Part model, mm, in its own coordinate system. A direction names the side the tool comes from. Give positions to 0.01 mm unless a question says otherwise; leave off trailing zeros. Write each loop counter-clockwise with the first axis right and the second up, starting at its lowest first coordinate (ties: lowest second). Pieces come first, ordered by that corner, then holes. Notation, with made-up numbers: (-26.5, -18.75) - (-12.5, -18.75) arc R19 ccw to (-12.5, 4.25) - close; hole circle Ø8 at (-22.75, -15). An arc over 180 degrees is marked (long way). Answer in a Markdown table with one row per item. Add a question column.
1. Band-saw the part on D-D on z = 2.7. Write the cut outline in (x, y), plus the area to 3 significant figures.
2. Probe line 1 along Z through (x, y) = (-7, -9.25); line 2 along Y through (x, z) = (-16, 3.4); line 3 along Y through (x, z) = (-13.25, 4.5). List the from-to ranges inside material, lowest first.
3. Band-saw the part on C-C on z = 1.2. Write the cut outline in (x, y), plus the area to 3 significant figures.
4. Band-saw the part on A-A on y = -5.5. Write the cut outline in (x, z).
5. Which spindle directions (+Z, -Z, +X, -X, +Y, -Y) get a long thin tool onto all of the face, cutting with end or side? Do faces 5 (the flat face through (-8, -10.7, 2)), 6 (the flat face through (-10, -5, 0)). Say none if no direction does.
6. Pull direction Y, two halves, no side cores. Call faces 1 (the flat face through (-9, 0, 2)), 2 (the flat face through (-20.377, -5, 2)), 3 (the flat face through (-8, -11, 2)), 4 (the flat face through (-10, -6, 4.7)): released by +Y, released by -Y, zero draft, split by the parting line, or undercut.
7. Band-saw the part on B-B on x = -2.75. Write the cut outline in (y, z).
8. Drop a flat-ended pin along its axis: pin 1 Ø0.6 at (y, z) = (-0.5, 2.5) entering from -X. Give the stop position or say it passes through.
Autodesk Inventor part; units mm, degrees
ref_plane "Work Plane1" through (-16.877, -0.4, 5) normal (-0.6428, 0, 0.766) x (0, -1, 0)
ref_plane "Work Plane2" through (-16.877, -0.4, 0) normal (-0.6428, 0, -0.766) x (0, -1, 0)
ref_plane "YZ Plane" through (0, 0, 0) normal (1, 0, 0) x (0, 1, 0)
sketch "Sketch1" plane through (0, 0, 0) normal (0, 0, 1) x (1, 0, 0)
  line L0 (0, -11) -> (-16.777, -11)
  line L1 (-16.777, -11) -> (-16.777, -10.7)
  line L2 (-16.777, -10.7) -> (0, -10.7)
  line L3 (0, -10.7) -> (0, -11)
  line L4 (0, -0.3) -> (-16.777, -0.3)
  line L5 (-16.777, -0.3) -> (-16.777, 0)
  line L6 (-16.777, 0) -> (0, 0)
  line L7 (0, 0) -> (0, -0.3)
  line L8 (-20.377, -8.65) -> (-20.777, -8.65)
  line L9 (-20.777, -8.65) -> (-20.777, -2.35)
  line L10 (-20.777, -2.35) -> (-20.377, -2.35)
  line L11 (-20.377, -2.35) -> (-20.377, -8.65)
  line L12 (-20.377, -8.65) -> (-16.777, -10.7)
  line L13 (-16.777, -11) -> (-20.777, -8.65)
  line L14 (-20.777, -2.35) -> (-16.777, 0)
  line L15 (-20.377, -2.35) -> (-16.777, -0.3)
  dimension "d0" = 0.3
  dimension "d2" = 10.4
  dimension "d3" = 0.4
  dimension "d4" = 4
  dimension "d21" = 20.777
  dimension "d22" = 6.3
extrude "Extrusion1" add sketch "Sketch1" along normal blind 5
sketch "Sketch2" plane through (-16.777, -10.7, 0) normal (0, 1, 0) x (1, 0, 0)
  line L0 (4.777, -3.6) -> (4.377, -3.6)
  line L1 (4.377, -3.6) -> (4.377, -1.4)
  line L2 (4.377, -1.4) -> (4.777, -1.4)
  line L3 (4.777, -1.4) -> (4.777, -3.6)
  line L4 (4.777, -3.6) -> (4.777, -5) construction
  line L5 (16.777, -5) -> (0, -5) construction
  line L6 (4.777, -1.4) -> (4.777, 0) construction
  line L7 (16.777, 0) -> (0, 0) construction
  line L8 (16.777, 0) -> (16.777, -5) construction
  dimension "d9" = 0.4
  dimension "d10" = 1.4
  dimension "d11" = 12
extrude "Extrusion2" add sketch "Sketch2" along normal blind 0.5
sketch "Sketch3" plane through (-16.777, -0.3, 0) normal (0, -1, 0) x (1, 0, 0)
  line L0 (4.777, 1.4) -> (4.377, 1.4)
  line L1 (4.377, 1.4) -> (4.377, 3.6)
  line L2 (4.377, 3.6) -> (4.777, 3.6)
  line L3 (4.777, 3.6) -> (4.777, 1.4)
  point P0 (16.777, 0)
extrude "Extrusion3" add sketch "Sketch3" along normal blind 0.5
sketch "Sketch4" plane through (0, -0.3, 0) normal (1, 0, 0) x (0, 0, -1)
  line L0 (0, -10.4) -> (-5, -10.4)
  line L1 (0, 0) -> (-5, 0)
  line L2 (-5, -10.4) -> (-4.7, -10.4)
  line L3 (-4.7, -10.4) -> (-4.7, 0)
  line L4 (-4.7, 0) -> (-5, 0)
  line L5 (-5, 0) -> (-5, -10.4)
  line L6 (0, 0) -> (-0.3, 0)
  line L7 (-0.3, 0) -> (-0.3, -10.4)
  line L8 (-0.3, -10.4) -> (0, -10.4)
  line L9 (0, -10.4) -> (0, 0)
  point P0 (0, 0.3)
  point P1 (-0.3, 0)
  dimension "d16" = 0.3
  dimension "d17" = 0.3
extrude "Extrusion4" add sketch "Sketch4" against normal up to next contours L0 L7 L1 L9 | L0 L5 L1 L3
fillet "Fillet1" radius 0.4 18 edges at (-20.777, -5.5, 0) (-18.777, -9.825, 0) (-18.777, -9.825, 5) (-20.777, -5.5, 5) (-18.777, -1.175, 0) (-18.777, -1.175, 5) (-8.3885, 0, 5) (-8.3885, 0, 0) (-8.3885, -11, 5) (-8.3885, -11, 0) (-8.3885, -10.7, 0.3) (-16.777, -10.7, 2.5) (-20.377, -8.65, 2.5) (-20.377, -2.35, 2.5) (-16.777, -0.3, 2.5) (-8.3885, -0.3, 0.3) (-8.3885, -0.3, 4.7) (-8.3885, -10.7, 4.7)
sketch "Sketch5" plane through (0, 0, 5) normal (0, 0, 1) x (1, 0, 0)
  line L0 (0, -0.4) -> (-16.6682, -0.4)
  line L1 (-16.877, -0.4) -> (-16.877, -10.7)
  line L2 (-16.6711, -10.7) -> (0, -10.7)
  line L3 (-20.377, -8.4211) -> (-20.377, -2.5789)
  point P0 (0, 0)
  dimension "d23" = 3.5
ref_plane "Work Plane1" through (-16.877, -0.4, 5) normal (-0.6428, 0, 0.766) x (0, -1, 0)
sketch "Sketch6" plane through (0, 0, 0) normal (0, 0, -1) x (-1, 0, 0)
  line L0 (16.877, -0.4) -> (16.877, -10.7)
  point P0 (0, 0)
ref_plane "Work Plane2" through (-16.877, -0.4, 0) normal (-0.6428, 0, -0.766) x (0, -1, 0)
sketch "Sketch7" plane through (-16.877, -0.4, 5) normal (-0.6428, 0, 0.766) x (0, -1, 0)
  line L0 (0.35, 0.6) -> (9.85, 0.6)
  line L1 (9.85, 0.6) -> (9.85, 0)
  line L2 (9.85, 0) -> (0.35, 0)
  line L3 (0.35, 0) -> (0.35, 0.6)
  line L4 (0, 0) -> (10.3, 0)
  line L5 (-0.4, 12.6714) -> (-0.4, -0.1805) construction
  line L6 (10.6, -0.1805) -> (10.6, 12.6714) construction
  line L7 (0.35, 0.6) -> (-0.4, 0.6) construction
  line L8 (9.85, 0.6) -> (10.6, 0.6) construction
  point P0 (-0.4, 9.7146)
  dimension "d26" = 9.5
  dimension "d27" = 0.6
extrude "Extrusion5" cut sketch "Sketch7" against normal blind 3
sketch "Sketch8" plane through (-16.877, -0.4, 0) normal (-0.6428, 0, -0.766) x (0, -1, 0)
  line L0 (9.85, -0.6) -> (0.35, -0.6)
  line L1 (0.35, -0.6) -> (0.35, 0)
  line L2 (0.35, 0) -> (9.85, 0)
  line L3 (9.85, 0) -> (9.85, -0.6)
  line L4 (0, 0) -> (10.3, 0)
  line L5 (0.35, 3.2139) -> (0.35, 2.6139)
  line L6 (9.85, 2.6139) -> (9.85, 3.2139)
  line L7 (10.6, -12.6714) -> (10.6, 0.1805)
  line L8 (-0.4, 0.1805) -> (-0.4, -12.6714)
  line L9 (0.35, -0.6) -> (-0.4, -0.6) construction
  line L10 (9.85, -0.6) -> (10.6, -0.6) construction
  point P0 (-0.4, -12.9285)
  dimension "d30" = 9.5
  dimension "d31" = 0.6
extrude "Extrusion6" cut sketch "Sketch8" against normal blind 3
sketch "Sketch9" plane through (0, 0, 0) normal (0, 0, -1) x (-1, 0, 0)
  circle A0 centre (19.977, -7.6) radius 0.4
  line L0 (19.977, -2.1106) -> (19.977, -5.2) construction
  line L1 (20.777, -8.65) -> (20.777, -2.35)
  circle A1 centre (19.977, -6.2) radius 0.4
  circle A2 centre (19.977, -4.8) radius 0.4
  circle A3 centre (19.977, -3.4) radius 0.4
  circle A4 centre (17.777, -7.6) radius 0.4
  line L2 (17.777, -0.9242) -> (17.777, -5.2) construction
  circle A5 centre (17.777, -6.2) radius 0.4
  circle A6 centre (17.777, -4.8) radius 0.4
  circle A7 centre (17.777, -3.4) radius 0.4
  circle A8 centre (17.777, -9) radius 0.4
  circle A9 centre (17.777, -2) radius 0.4
  line L3 (19.977, -8) -> (19.977, -8.65) construction
  line L4 (20.777, -2.35) -> (16.777, 0)
  line L5 (20.777, -2.35) -> (20.777, -8.65)
  line L6 (20.777, -5.5) -> (17.4188, -5.5)
  line L7 (19.977, -5.5) -> (19.977, -5.8) construction
  line L8 (19.977, -5.8) -> (19.977, -8) construction
  line L9 (19.977, -5.2) -> (19.977, -5.5) construction
  line L10 (17.777, -5.8) -> (17.777, -10.129) construction
  line L11 (17.777, -5.5) -> (17.777, -5.8) construction
  line L12 (17.777, -5.2) -> (17.777, -5.5) construction
  line L13 (18.877, -9.1995) -> (18.877, -2.1819) construction
  circle A10 centre (18.877, -6.9) radius 0.4
  circle A11 centre (18.877, -5.5) radius 0.4
  circle A12 centre (18.877, -4.1) radius 0.4
  circle A13 centre (18.877, -2.7) radius 0.4
  circle A14 centre (18.877, -8.3) radius 0.4
  point P0 (0, 0)
  dimension "d35" = 0.8
  dimension "d34" = 0.8
  dimension "d36" = 1.4
  dimension "d37" = 1.4
  dimension "d38" = 1.4
  dimension "d39" = 0.8
  dimension "d40" = 1.4
  dimension "d41" = 1.4
  dimension "d42" = 1.4
  dimension "d43" = 1.4
  dimension "d44" = 1.4
  dimension "d45" = 6.3
  dimension "d46" = 3.15
  dimension "d47" = 1.4
  dimension "d48" = 1.4
  dimension "d49" = 1.4
  dimension "d51" = 1.4
  dimension "d52" = 1.1
  dimension "d53" = 1.1
extrude "Extrusion7" cut sketch "Sketch9" against normal blind 0.2
sketch "Sketch10" plane through (0, 0, 5) normal (0, 0, 1) x (1, 0, 0)
  circle A0 centre (-17.777, -9) radius 0.4
  circle A1 centre (-17.777, -7.6) radius 0.4
  circle A2 centre (-17.777, -6.2) radius 0.4
  circle A3 centre (-17.777, -4.8) radius 0.4
  circle A4 centre (-17.777, -3.4) radius 0.4
  circle A5 centre (-17.777, -2) radius 0.4
  circle A6 centre (-18.877, -2.7) radius 0.4
  circle A7 centre (-18.877, -4.1) radius 0.4
  circle A8 centre (-18.877, -5.5) radius 0.4
  circle A9 centre (-18.877, -6.9) radius 0.4
  circle A10 centre (-18.877, -8.3) radius 0.4
  circle A11 centre (-19.977, -7.6) radius 0.4
  circle A12 centre (-19.977, -6.2) radius 0.4
  circle A13 centre (-19.977, -4.8) radius 0.4
  circle A14 centre (-19.977, -3.4) radius 0.4
  point P0 (0, 0)
  point P1 (-20.377, -7.6)
  point P2 (-20.377, -6.2)
  point P3 (-20.377, -4.8)
  point P4 (-20.377, -3.4)
extrude "Extrusion8" cut sketch "Sketch10" against normal blind 0.2
equation "\"d17\" = d16"
equation "\"d43\" = d36"
equation "\"d44\" = d36"
equation "\"d46\" = 0.5 * d45"
properties part number "np2_headstage_box"
Values:
| question | item | result |
|---|---|---|
| 1 | outline | (-20.78, -8.65) - (-16.78, -11) - (0, -11) - (0, -10.7) - (-12, -10.7) - (-12, -10.2) - (-12.4, -10.2) - (-12.4, -10.7) - (-16.67, -10.7) arc R0.4 cw to (-16.87, -10.65) - (-20.17, -8.77) arc R0.4 cw to (-20.38, -8.42) - (-20.38, -2.58) arc R0.4 cw to (-20.17, -2.23) - (-16.87, -0.35) arc R0.4 cw to (-16.67, -0.3) - (-12.4, -0.3) - (-12.4, -0.8) - (-12, -0.8) - (-12, -0.3) - (0, -0.3) - (0, 0) - (-16.78, 0) - (-20.78, -2.35) - close |
| 1 | area | 15.0 mm² |
| 2 | line 1 | z = 0 to 0.3, 4.7 to 5 |
| 2 | line 2 | y = -11 to -10.7, -0.3 to 0 |
| 2 | line 3 | y = -11 to -10.65, -0.35 to 0 |
| 3 | outline | (-20.78, -8.65) - (-16.78, -11) - (0, -11) - (0, -10.7) - (-16.67, -10.7) arc R0.4 cw to (-16.87, -10.65) - (-20.17, -8.77) arc R0.4 cw to (-20.38, -8.42) - (-20.38, -2.58) arc R0.4 cw to (-20.17, -2.23) - (-16.87, -0.35) arc R0.4 cw to (-16.67, -0.3) - (0, -0.3) - (0, 0) - (-16.78, 0) - (-20.78, -2.35) - close |
| 3 | area | 14.6 mm² |
| 4 | outline | (-20.78, 0.4) arc R0.4 ccw to (-20.38, 0) - (-19.28, 0) - (-19.28, 0.2) - (-18.48, 0.2) - (-18.48, 0) - (-16.88, 0) - (-16.63, 0.3) - (-20.38, 0.3) - (-20.38, 4.7) - (-16.63, 4.7) - (-16.88, 5) - (-18.48, 5) - (-18.48, 4.8) - (-19.28, 4.8) - (-19.28, 5) - (-20.38, 5) arc R0.4 ccw to (-20.78, 4.6) - close; (-16.09, 0) - (0, 0) - (0, 0.3) - (-15.84, 0.3) - close; (-16.09, 5) - (-15.84, 4.7) - (0, 4.7) - (0, 5) - close |
| 5 | face 5 | none |
| 5 | face 6 | -Z, +X, -X, +Y, -Y |
| 6 | face 1 | released by +Y |
| 6 | face 2 | undercut |
| 6 | face 3 | released by -Y |
| 6 | face 4 | undercut |
| 7 | outline | (-11, 0.4) arc R0.4 ccw to (-10.6, 0) - (-0.4, 0) arc R0.4 ccw to (0, 0.4) - (0, 4.6) arc R0.4 ccw to (-0.4, 5) - (-10.6, 5) arc R0.4 ccw to (-11, 4.6) - close; hole (-10.7, 0.7) arc R0.4 ccw to (-10.3, 0.3) - (-0.7, 0.3) arc R0.4 ccw to (-0.3, 0.7) - (-0.3, 4.3) arc R0.4 ccw to (-0.7, 4.7) - (-10.3, 4.7) arc R0.4 ccw to (-10.7, 4.3) - close |
| 8 | pin 1 | stops at x = -18.14 |
